Can you work these out from the model? Positions are in its coordinate system, mm. Give positions to 0.01 mm unless a question says otherwise; leave off trailing zeros. Order: outer loops, then holes, each group sorted by start corner. A loop starts at its lowest first (then second) coordinate and runs counter-clockwise, first axis right, second up. Notation, with made-up numbers: (59.25, 73.5) - (115.25, 73.5) arc R18 ccw to (115.25, 91.5) - close; hole circle Ø10 at (-6.75, 34.25). An arc over 180 degrees is marked (long way). Return JSON: item names as keys, results as strings.
```python
from build123d import *

# Parameters (mm, degrees)
SKETCH1_W               = 76.2
SKETCH1_H               = 76.2
SKETCH1_R               = 25.4
BOSS_EXTRUDE1_DEPTH     = 1.5875
SKETCH2_R               = 3.302
CUT_EXTRUDE1_DEPTH      = 3.175
MIRROR2_COPY_1_SKETCH_R = 3.302
MIRROR2_COPY_1_DEPTH    = 3.175
SKETCH9_W               = 4.7625
SKETCH9_H               = 53.34
CUT_EXTRUDE3_DEPTH      = 2.5875


with BuildPart() as part:
    # Sketch1 → Boss-Extrude1 (new body)
    with BuildSketch(Plane.XY):
        Rectangle(SKETCH1_W, SKETCH1_H)
        Circle(SKETCH1_R, mode=Mode.SUBTRACT)
    extrude(amount=BOSS_EXTRUDE1_DEPTH)

    # Sketch2 → Cut-Extrude1 (cut)
    with BuildSketch(Plane.XY.offset(1.5875)):
        with Locations((-31.75, 31.75)):
            Circle(SKETCH2_R)
    cut_extrude1 = extrude(amount=-CUT_EXTRUDE1_DEPTH, mode=Mode.SUBTRACT)

    # Mirror1: Cut-Extrude1 across plane
    add(cut_extrude1.mirror(Plane(origin=(0, 0, 0), x_dir=(0, 0, 1), z_dir=(1, 0, 0))), mode=Mode.SUBTRACT)

    # Mirror2: Cut-Extrude1 across plane
    add(cut_extrude1.mirror(Plane.ZX), mode=Mode.SUBTRACT)

    # Mirror2 copy 1 sketch → Mirror2 copy 1 (cut)
    with BuildSketch(Plane(origin=(0, 0, 1.5875), x_dir=(-1, 0, 0), z_dir=(0, 0, 1))):
        with Locations((-31.75, 31.75)):
            Circle(MIRROR2_COPY_1_SKETCH_R)
    extrude(amount=-MIRROR2_COPY_1_DEPTH, mode=Mode.SUBTRACT)

    # Sketch9 → Cut-Extrude3 (cut, through all)
    with BuildSketch(Plane.XY.offset(1.5875)):
        with Locations((-35.71875, 0)):
            Rectangle(SKETCH9_W, SKETCH9_H)
    cut_extrude3 = extrude(amount=-CUT_EXTRUDE3_DEPTH, mode=Mode.SUBTRACT)

    # Mirror3: Cut-Extrude3 across plane
    add(cut_extrude3.mirror(Plane(origin=(0, 0, 0), x_dir=(0, 0, 1), z_dir=(1, 0, 0))), mode=Mode.SUBTRACT)


solid = part.part
```
1. Suppose I cut it at C-C (z = 0.6). List the corners of the cut face in (x, y) for me.
Checks:
{"outline": "(-38.1, -38.1) - (38.1, -38.1) - (38.1, -26.67) - (33.34, -26.67) - (33.34, 26.67) - (38.1, 26.67) - (38.1, 38.1) - (-38.1, 38.1) - (-38.1, 26.67) - (-33.34, 26.67) - (-33.34, -26.67) - (-38.1, -26.67) - close; hole circle Ø6.6 at (-31.75, -31.75); hole circle Ø6.6 at (-31.75, 31.75); hole circle Ø50.8 at (0, 0); hole circle Ø6.6 at (31.75, -31.75); hole circle Ø6.6 at (31.75, 31.75)"}
2. For pin 1 Ø0.5 at (y, z) = (-8.5, 1) entering from -X, with a flat end and sliding along its axis, tell me the tip position at first contact or that it passes through.
Checks:
{"pin 1": "x = -33.34"}
3. If I drill on L1, parallel to X at y = -31.75, z = 0.6; L2, parallel to X at y = 0.5, z = 0.75; L3, parallel to Y at x = 0, z = 1.15, over which ranges is the centre line in solid material (lowest first)? Write a range as [from, to].
Checks:
{"L1": "[-38.1, -35.05], [-28.45, 28.45], [35.05, 38.1]", "L2": "[-33.34, -25.4], [25.4, 33.34]", "L3": "[-38.1, -25.4], [25.4, 38.1]"}
4. Suppose I cut it at D-D (y = 0). List the corners of the cut face in (x, z) for me, plus the area to 3 significant figures.
Checks:
{"outline": "(-33.34, 0) - (-25.4, 0) - (-25.4, 1.59) - (-33.34, 1.59) - close; (25.4, 0) - (33.34, 0) - (33.34, 1.59) - (25.4, 1.59) - close", "area": "25.2 mm^2"}
5. Thinking about a two-plate mould opening in Y: for faces 1 (the face through (25, 9, 0)), 2 (the face through (-5.506, -24.796, 0.783)), 3 (the face through (30.23, 28.82, 0.8)), which applies, +Y half, -Y half, draft (parallel to the pull), parting line (faces both ways), or undercut?
Checks:
{"face 1": "draft", "face 2": "undercut", "face 3": "undercut"}
6. Suppose I cut it at A-A (y = 31.75). List the corners of the cut face in (x, z) for me, plus the area to 4 significant figures.
Checks:
{"outline": "(-38.1, 0) - (-35.05, 0) - (-35.05, 1.59) - (-38.1, 1.59) - close; (-28.45, 0) - (28.45, 0) - (28.45, 1.59) - (-28.45, 1.59) - close; (35.05, 0) - (38.1, 0) - (38.1, 1.59) - (35.05, 1.59) - close", "area": "100.0 mm^2"}
